Geometry: see drawing. Coordinates: mm, zero at the bounding-box minimum. A direction names the side the tool comes from. Round coordinates to 2 decimals unless told otherwise and drop trailing zeros. Loops run counter-clockwise (first coordinate to the right, second up) from the corner with the lowest first, then second, coordinate; pieces in that order, holes last.
(1) Draft query along Z for the marked faces 1, 2 and 3. Return one class per face: released by +Z, released by -Z, zero draft, split by the parting line, or undercut.
(2) Cut plane B-B, the plane y = 5. Output: boundary loops of the cut face in (x, z) (1 decimal).
(3) Line query: line 1 (Z direction, x = 5.25, y = 4.5) (1 decimal); line 2 (Z direction, x = 7, y = 3.5) (1 decimal); line 3 (X direction, y = 3, z = 4) (1 decimal). Output: solid intervals per line, ascending.
(4) Cut plane A-A, the plane y = 8. Output: boundary loops of the cut face in (x, z) (1 decimal).
(5) Access query for the marked faces 4 and 5. Directions: +Z, -Z, +X, -X, +Y, -Y. A direction counts if a zero-diameter tool reaches every point of the face in a straight line with its end or side. Return the directions, or none.
(6) First-contact query: pin 1 Ø2 at (y, z) = (2.5, 1) entering from -X. Flat tip, straight axial feed; report the tip coordinate or a pass-through.
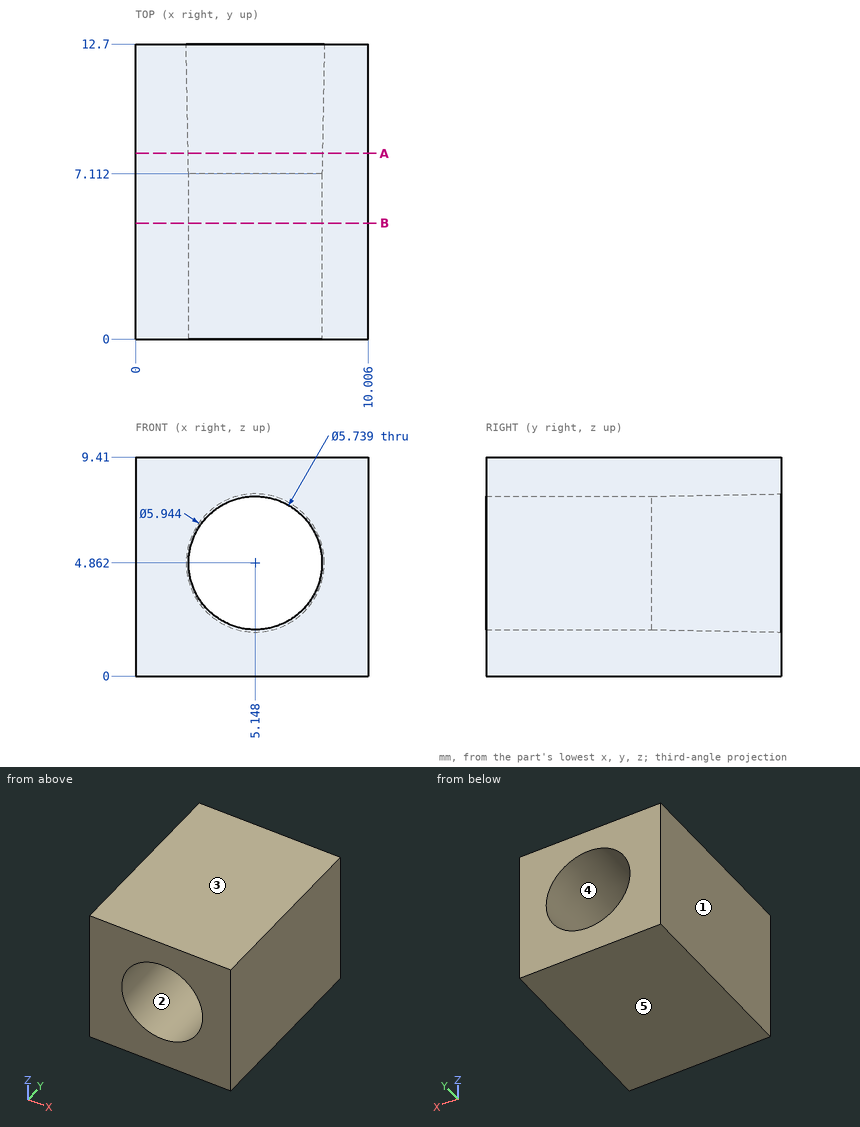
Reported:
1. face 1: zero draft
1. face 2: undercut
1. face 3: released by +Z
2. outline: (0, 0) - (10, 0) - (10, 9.4) - (0, 9.4) - close; hole circle Ø5.7 at (5.1, 4.9)
3. line 1: z = 0 to 2, 7.7 to 9.4
3. line 2: z = 0 to 2.7, 7.1 to 9.4
3. line 3: x = 0 to 2.4, 7.9 to 10
4. outline: (0, 0) - (10, 0) - (10, 9.4) - (0, 9.4) - close; hole circle Ø5.8 at (5.1, 4.9)
5. face 4: +Y
5. face 5: -Z, +X, -X, +Y, -Y
6. pin 1: stops at x = 0
